The listing builds one solid part. Answer for the finished solid, in the listing's coordinates (mm). A direction names the side the tool comes from. Give positions to 0.01 mm unless a question says otherwise; leave off trailing zeros. Loops run counter-clockwise (first coordinate to the right, second up) from the corner with the lowest first, then second, coordinate; pieces in that order, holes last. Notation, with made-up numbers: (-25, 85) - (22, 85) arc R18 cw to (22, 119) - close; hole circle Ø1 at (30.5, 75.25). An arc over 180 degrees is marked (long way). One line per item, written item: value. Start each with the question number.
from build123d import *

# Parameters (mm, degrees)
SKETCH1_R                  = 25.4
SKETCH1_R_2                = 22.86
TUBE_CONNECTION_RING_DEPTH = 19.05
SKETCH6_R                  = 2.286
SCREW_HOLE_DEPTH           = 19.05
NUT_PRESS_FIT_HOLE_START   = -11.059647
NUT_PRESS_FIT_HOLE_DEPTH   = 3.81
CIRPATTERN1_COUNT          = 4
SCREW_HOLE_CHAMFER_SIZE    = 2.884664172
SCREW_HOLE_CHAMFER_SIZE_2  = 2.54
SKETCH12_R                 = 27.6225
SKETCH12_R_2               = 3.302
TOP_PLATE_DEPTH            = 3.81
HINGE_HOLE_DEPTH           = 19.05
HINGE_HOLE_CUT_REACH       = 66.384
SKETCH14_R                 = 2.54


with BuildPart() as part:
    # Sketch1 → tube_connection_ring (new body)
    # profile 1 of 5: a face of its own
    with BuildSketch(Plane(origin=(0, 0, 0), x_dir=(1, 0, 0), z_dir=(0, 1, 0))):
        with Locations(Location((0, 0, 0), (0, 0, 90))):
            Circle(SKETCH1_R)
        Circle(SKETCH1_R_2, mode=Mode.SUBTRACT)
    # profile 2 of 5: a face of its own
    with BuildSketch(Plane(origin=(0, 0, 0), x_dir=(1, 0, 0), z_dir=(0, 1, 0))):
        with BuildLine():
            ThreePointArc((22.86, 0), (22.633970791, 3.206706444), (21.960352912, 6.35))
            Line((21.960352912, 6.35), (14.340352912, 3.175))
            Line((14.340352912, 3.175), (14.340352912, -3.175))
            Line((14.340352912, -3.175), (21.960352912, -6.35))
            ThreePointArc((21.960352912, -6.35), (22.633970791, -3.206706444), (22.86, 0))
        make_face()
    # profile 3 of 5: a face of its own
    with BuildSketch(Plane(origin=(0, 0, 0), x_dir=(1, 0, 0), z_dir=(0, 1, 0))):
        with BuildLine():
            ThreePointArc((-6.35, -21.960352912), (0, -22.86), (6.35, -21.960352912))
            Line((6.35, -21.960352912), (3.175, -14.340352912))
            Line((3.175, -14.340352912), (-3.175, -14.340352912))
            Line((-3.175, -14.340352912), (-6.35, -21.960352912))
        make_face()
    # profile 4 of 5: a face of its own
    with BuildSketch(Plane(origin=(0, 0, 0), x_dir=(1, 0, 0), z_dir=(0, 1, 0))):
        with BuildLine():
            Line((-14.340352912, 3.175), (-21.960352912, 6.35))
            ThreePointArc((-21.960352912, 6.35), (-22.86, 0), (-21.960352912, -6.35))
            Line((-21.960352912, -6.35), (-14.340352912, -3.175))
            Line((-14.340352912, -3.175), (-14.340352912, 3.175))
        make_face()
    # profile 5 of 5: a face of its own
    with BuildSketch(Plane(origin=(0, 0, 0), x_dir=(1, 0, 0), z_dir=(0, 1, 0))):
        with BuildLine():
            Line((3.175, 14.340352912), (6.35, 21.960352912))
            ThreePointArc((6.35, 21.960352912), (0, 22.86), (-6.35, 21.960352912))
            Line((-6.35, 21.960352912), (-3.175, 14.340352912))
            Line((-3.175, 14.340352912), (3.175, 14.340352912))
        make_face()
    extrude(amount=TUBE_CONNECTION_RING_DEPTH)

    # Sketch6 → screw_hole (cut)
    with BuildSketch(Plane(origin=(25.4, 0, 0), x_dir=(0, 0, -1), z_dir=(1, 0, 0))):
        with Locations((0, 9.525)):
            Circle(SKETCH6_R)
    screw_hole = extrude(amount=-SCREW_HOLE_DEPTH, mode=Mode.SUBTRACT)

    # Sketch11 → nut_press_fit_hole (cut)
    with BuildSketch(Plane(origin=(25.4, 0, 0), x_dir=(0, 0, -1), z_dir=(1, 0, 0)).offset(NUT_PRESS_FIT_HOLE_START)):
        Polygon((0, 4.09906217), (4.699, 6.812031085), (4.699, 12.237968915), (0, 14.95093783), (-4.699, 12.237968915), (-4.699, 6.812031085), align=None)
    nut_press_fit_hole = extrude(amount=NUT_PRESS_FIT_HOLE_DEPTH, mode=Mode.SUBTRACT)

    # CirPattern1: screw_hole, nut_press_fit_hole ×4 about axis
    cirpattern1_axis = Axis((0, 0, 0), (0, 1, 0))
    add([screw_hole.rotate(cirpattern1_axis, i * 360 / CIRPATTERN1_COUNT) for i in range(1, CIRPATTERN1_COUNT)], mode=Mode.SUBTRACT)
    add([nut_press_fit_hole.rotate(cirpattern1_axis, i * 360 / CIRPATTERN1_COUNT) for i in range(1, CIRPATTERN1_COUNT)], mode=Mode.SUBTRACT)

    # screw_hole_chamfer
    # the kernel refuses this chamfer: 2.884664172, 2.54 mm, written as the material it adds along each edge
    with BuildSketch(Plane(origin=(-6.35, 0, -21.960352912), x_dir=(-0.9446263547307573, 0, 0.32814790864499105), z_dir=(0, 1, 0)), Plane(origin=(-21.960352912, 0, 6.35), x_dir=(0.3281479086449895, 0, 0.944626354730758), z_dir=(0, 1, 0)), Plane(origin=(6.35, 0, 21.960352912), x_dir=(0.9446263547307586, 0, -0.32814790864498755), z_dir=(0, 1, 0)), Plane(origin=(21.960352912, 0, -6.35), x_dir=(-0.3281479086449886, 0, -0.9446263547307582), z_dir=(0, 1, 0))) as screw_hole_chamfer_piece_1:
        with BuildLine():
            Line((2.415733057, 0), (-SCREW_HOLE_CHAMFER_SIZE * 0.0604120669079, SCREW_HOLE_CHAMFER_SIZE * 0.998173522936))
            Line((-SCREW_HOLE_CHAMFER_SIZE * 0.0604120669079, SCREW_HOLE_CHAMFER_SIZE * 0.998173522936), (0, 0))
            ThreePointArc((0, 0), (1.246430784, -0.031900132), (2.415733057, 0))
        make_face()
    extrude(amount=19.05)
    with BuildSketch(Plane(origin=(-21.960352912, 0, -6.35), x_dir=(0.9230769230769231, 0, 0.38461538461538464), z_dir=(0, 1, 0)), Plane(origin=(-6.35, 0, 21.960352912), x_dir=(0.3846153846153849, 0, -0.9230769230769229), z_dir=(0, 1, 0)), Plane(origin=(21.960352912, 0, 6.35), x_dir=(-0.9230769230769229, 0, -0.3846153846153849), z_dir=(0, 1, 0))) as screw_hole_chamfer_piece_2:
        with BuildLine():
            Line((SCREW_HOLE_CHAMFER_SIZE_2, 0), (-0.146371443, 2.686371443))
            ThreePointArc((-0.146371443, 2.686371443), (-0.11503611, 1.383925534), (0, 0))
            Line((0, 0), (SCREW_HOLE_CHAMFER_SIZE_2, 0))
        make_face()
    extrude(amount=19.05)
    with BuildSketch(Plane(origin=(6.35, 0, -21.960352912), x_dir=(0.9426351264301257, 0, 0.3338248319404367), z_dir=(0, 1, 0))) as screw_hole_chamfer_piece_3:
        with BuildLine():
            Line((2.690356134, 0), (-SCREW_HOLE_CHAMFER_SIZE_2 * 0.0544059729896, -SCREW_HOLE_CHAMFER_SIZE_2 * 0.99851889822))
            Line((-SCREW_HOLE_CHAMFER_SIZE_2 * 0.0544059729896, -SCREW_HOLE_CHAMFER_SIZE_2 * 0.99851889822), (0, 0))
            ThreePointArc((0, 0), (1.388134451, 0.039571914), (2.690356134, 0))
        make_face()
    extrude(amount=19.05)

    # Sketch12 → top_plate (add)
    with BuildSketch(Plane(origin=(0, 19.05, 0), x_dir=(1, 0, 0), z_dir=(0, 1, 0))):
        with Locations(Location((0, 0, 0), (0, 0, 90))):
            Circle(SKETCH12_R)
        with Locations(Location((0, 0, 0), (0, 0, 90))):
            Circle(SKETCH12_R_2, mode=Mode.SUBTRACT)
    extrude(amount=TOP_PLATE_DEPTH)

    # Sketch13 → hinge_hole (add)
    with BuildSketch(Plane(origin=(0, 22.86, 0), x_dir=(1, 0, 0), z_dir=(0, 1, 0))):
        with BuildLine():
            ThreePointArc((24.529828908, -12.7), (25.666241564, -10.210119991), (26.550670542, -7.62))
            Line((26.550670542, -7.62), (8.89, -7.62))
            Line((8.89, -7.62), (8.89, 0))
            Line((8.89, 0), (6.35, 0))
            ThreePointArc((6.35, 0), (0, -6.35), (-6.35, 0))
            Line((-6.35, 0), (-8.89, 0))
            Line((-8.89, 0), (-8.89, -7.62))
            Line((-8.89, -7.62), (-26.550670542, -7.62))
            ThreePointArc((-26.550670542, -7.62), (-25.666241564, -10.210119991), (-24.529828908, -12.7))
            Line((-24.529828908, -12.7), (24.529828908, -12.7))
        make_face()
    extrude(amount=HINGE_HOLE_DEPTH)

    # Sketch14 → hinge_hole_cut (cut, up to next)
    with BuildSketch(Plane.XY.offset(12.7), mode=Mode.PRIVATE) as hinge_hole_cut_sk1:
        with Locations((18.424251671, 31.75)):
            Circle(SKETCH14_R)
    hinge_hole_cut_tool1 = extrude(hinge_hole_cut_sk1.sketch, amount=-HINGE_HOLE_CUT_REACH, mode=Mode.PRIVATE) & part.part
    # Sketch14 → hinge_hole_cut (cut, up to next)
    with BuildSketch(Plane.XY.offset(12.7), mode=Mode.PRIVATE) as hinge_hole_cut_sk2:
        with Locations((-18.424251671, 31.75)):
            Circle(SKETCH14_R)
    hinge_hole_cut_tool2 = extrude(hinge_hole_cut_sk2.sketch, amount=-HINGE_HOLE_CUT_REACH, mode=Mode.PRIVATE) & part.part
    add(hinge_hole_cut_tool1.solids().sort_by_distance((18.424252, 31.75, 12.7))[0], mode=Mode.SUBTRACT)
    add(hinge_hole_cut_tool2.solids().sort_by_distance((-18.424252, 31.75, 12.7))[0], mode=Mode.SUBTRACT)


solid = part.part
1. Determine the mould class of faces 4 (the flat face through (8.1, 19.05, -24.4)), 5 (the cylindrical face through (-0.99, 20.93, -3.15)), 6 (the flat face through (1.794, 13.915, -16.219)) for opening direction Y: released by +Y, released by -Y, zero draft, split by the parting line, or undercut.
2. Find the intervals of material crossed by L1, parallel to X at y = 18, z = -18; L2, parallel to Y at x = -23, z = 0; L3, parallel to Z at x = 15.5, y = 4.5, in increasing order. Write a range as [from, to].
3. A cutting plane is placed at D-D (x = 11). Determine the outline of the cut face in (y, z).
4. A cutting plane is placed at A-A (y = 31.75). Give the number of separate pieces and of enclosed holes in the cut face, plus the area to 3 significant figures.
5. A cutting plane is placed at C-C (y = 21.5). Determine the outline of the cut face in (x, z) (1 decimal), plus the area to 3 significant figures.
6. For faces 1 (the flat face through (1.86, 13.877, 16.219)), 2 (the flat face through (20.329, 9.392, 7.105)), 3 (the flat face through (0, 32, 12.7)), determine the directions among +Z, -Z, +X, -X, +Y, -Y from which every point of the face is accessible in a straight line to the end or side of a thin tool.
7. Flat-ended cylindrical pins translate along their axes: pin 1 (7.5 mm diameter, centred on y = 10.5, z = 2, fed in from +X); pin 2 (3 mm diameter, centred on x = -1.5, y = 9, fed in from +Z); pin 3 (1.5 mm diameter, centred on x = 7.5, y = 21, fed in from +Z); pin 4 (4 mm diameter, centred on x = 0, y = 9.525, fed in from +Z). Find the tip coordinate at first contact, or state that the pin passes through.
8. A cutting plane is placed at B-B (z = 11). Determine the outline of the cut face in (x, y), plus the area to 3 significant figures.
Results below:
1. face 4: released by -Y
1. face 5: zero draft
1. face 6: undercut
2. L1: x = [-17.92, -14.09], [-4.7, 4.7], [14.09, 17.92]
2. L2: y = [0, 7.24], [11.81, 22.86]
2. L3: z = [-20.12, -16.8], [-3.66, -0.69], [0.69, 3.66], [16.8, 20.12]
3. outline: (0, -22.89) - (19.05, -22.89) - (19.05, -25.34) - (22.86, -25.34) - (22.86, 7.62) - (41.91, 7.62) - (41.91, 12.7) - (22.86, 12.7) - (22.86, 25.34) - (19.05, 25.34) - (19.05, 22.89) - (0, 22.89) - (0, 20.04) - (19.05, 20.04) - (19.05, -20.04) - (0, -20.04) - close
4. separate pieces: 3
4. enclosed holes: 0
4. area: 281 mm^2
5. outline: circle Ø55.2 at (0, 0); hole circle Ø6.6 at (0, 0)
5. area: 2,360 mm^2
6. face 1: none
6. face 2: -Y
6. face 3: +Z, +X, -X, +Y
7. pin 1: stops at x = 25.4
7. pin 2: stops at z = 25.37
7. pin 3: stops at z = 26.79
7. pin 4: passes through
8. outline: (-25.34, 19.05) - (-22.89, 19.05) - (-22.89, 0) - (-20.04, 0) - (-20.04, 19.05) - (20.04, 19.05) - (20.04, 0) - (22.89, 0) - (22.89, 19.05) - (25.34, 19.05) - (25.34, 41.91) - (-25.34, 41.91) - close; hole circle Ø5.08 at (-18.42, 31.75); hole circle Ø5.08 at (18.42, 31.75)
8. area: 1,230 mm^2
